Build history of the part. All positions in model axes, mm. Round coordinates to 2 decimals unless told otherwise and drop trailing zeros. Loops run counter-clockwise (first coordinate to the right, second up) from the corner with the lowest first, then second, coordinate; pieces in that order, holes last. Notation, with made-up numbers: (21, 26) - (49, 26) arc R23 cw to (49, 52) - close; hole circle Ø10 at (14, 38.25). An arc over 180 degrees is marked (long way). Use a Markdown table: item, result.
from build123d import *

# Parameters (mm, degrees)
F0_R     = 1.5621
F1_DEPTH = 33.02
F2_R     = 2.54
F3_DEPTH = 1.905


# Not quite as in the source:
# - a fillet or chamfer that OpenCascade refuses, or shapes differently, is made with other operations: its cross-section is extruded or revolved along the edge and cut away or added


with BuildPart() as f1:
    # F0 (on Front) → F1 (new body)
    with BuildSketch(Plane.XZ):
        with Locations((10.1929502562, 6.33663591)):
            Circle(F0_R)
    extrude(amount=F1_DEPTH)

    # F2 (on face) → F3 (join)
    with BuildSketch(Plane.XZ.offset(33.02)):
        with Locations((10.1929502562, 6.33663591)):
            Circle(F2_R)
    extrude(amount=F3_DEPTH)

    # F4: fillet of radius 2.54 on 1 edges, made by hand

    # F4_s1 → F4_t2 (revolve, cut)
    with BuildSketch(Plane.XY.offset(6.33663591)):
        with BuildLine():
            ThreePointArc((12.7329502562, -33.02), (11.829031818, -34.3930463142), (10.2736058313, -34.925))
            Line((10.2736058313, -34.925), (12.7329502562, -34.925))
            Line((12.7329502562, -34.925), (12.7329502562, -33.02))
        make_face()
    revolve(axis=Axis((10.1929502562, -34.925, 6.33663591), (0, -1, 0)), mode=Mode.SUBTRACT)


solid = f1.part
Q1. Probe line 1 (X direction, y = -31, z = 6.4); line 2 (Z direction, x = 10.3, y = -11); line 3 (Y direction, x = 11.4, z = 7.45). List the from-to ranges inside material, lowest first.
Results found:
| item | result |
|---|---|
| line 1 | x = 8.63 to 11.75 |
| line 2 | z = 4.78 to 7.9 |
| line 3 | y = -34.39 to -33.02 |
Q2. Pull direction Y, two halves, no side cores. Call faces 1 (the face through (8.632, -16.279, 6.405)), 2 (the face through (11, -33.02, 8)): pulls with the +Y half, pulls with the -Y half, needs draft (parallel to the pull), parting line crosses it, or undercut.
Results found:
| item | result |
|---|---|
| face 1 | needs draft |
| face 2 | pulls with the +Y half |
Q3. Cut at A-A, the plane y = -25.5. List the corners of the cut face in (x, z), plus the area to 3 significant figures.
Results found:
| item | result |
|---|---|
| outline | circle Ø3.12 at (10.19, 6.34) |
| area | 7.67 mm2 |
Q4. Drop flat-ended pins along their axis: pin 1 (1.5 mm diameter, centred on y = -27.5, z = 5, fed in from -X); pin 2 (3 mm diameter, centred on x = 10, y = -17.5, fed in from +Z); pin 3 (1 mm diameter, centred on x = 10, z = 7.5, fed in from -Y). Give the stop position or say it passes through.
Results found:
| item | result |
|---|---|
| pin 1 | stops at x = 8.75 |
| pin 2 | stops at z = 7.9 |
| pin 3 | stops at y = -34.85 |
